from build123d import *

# Parameters (mm, degrees)
SKETCH1_R           = 2
BOSS_EXTRUDE1_DEPTH = 5
SKETCH2_R           = 4
CUT_EXTRUDE1_DEPTH  = 2
SKETCH3_R           = 11
SKETCH3_R_2         = 1.901621635
BOSS_EXTRUDE2_DEPTH = 12


with BuildPart() as part:
    # Sketch1 → Boss-Extrude1 (new body)
    with BuildSketch(Plane(origin=(0, 0, 0), x_dir=(1, 0, 0), z_dir=(0, 1, 0))):
        Polygon((0, 49), (0, 0), (49, 0), (49, 34), (34, 34), (34, 49), align=None)
        with Locations((15, 10.96347032)):
            Circle(SKETCH1_R, mode=Mode.SUBTRACT)
        with Locations((15, 25.96347032)):
            Circle(SKETCH1_R, mode=Mode.SUBTRACT)
        with Locations((15, 40.96347032)):
            Circle(SKETCH1_R, mode=Mode.SUBTRACT)
    extrude(amount=BOSS_EXTRUDE1_DEPTH)

    # Sketch2 → Cut-Extrude1 (cut)
    with BuildSketch(Plane(origin=(0, 5, 0), x_dir=(1, 0, 0), z_dir=(0, 1, 0))):
        with Locations((15, 40.96347032)):
            Circle(SKETCH2_R)
        with Locations((15, 10.96347032)):
            Circle(SKETCH2_R)
    extrude(amount=-CUT_EXTRUDE1_DEPTH, mode=Mode.SUBTRACT)

    # Sketch3 → Boss-Extrude2 (add)
    with BuildSketch(Plane(origin=(0, 5, 0), x_dir=(1, 0, 0), z_dir=(0, 1, 0))):
        with Locations((15, 25.96347032)):
            Circle(SKETCH3_R)
        with Locations((15, 25.96347032)):
            Circle(SKETCH3_R_2, mode=Mode.SUBTRACT)
    extrude(amount=BOSS_EXTRUDE2_DEPTH)


solid = part.part
The model under review builds one solid part; all positions refer to its coordinate system, in mm. A direction names the side the tool comes from. Round coordinates to 2 decimals unless told otherwise and drop trailing zeros. Order: outer loops, then holes, each group sorted by start corner. A loop starts at its lowest first (then second) coordinate and runs counter-clockwise, first axis right, second up. Notation, with made-up numbers: (-22.5, 78.5) -> (11.5, 78.5) arc R21 ccw to (11.5, 102.5) -> close; hole circle Ø11 at (62, -21.75). An arc over 180 degrees is marked (long way). Use CSV: the item, a comma, the result in double quotes. Start each with the question number.
(1) Wall thickness on probe 1 along Z at (x, y) = (15, 3.6); probe 2 along Z at (x, y) = (15, 1.2); probe 3 along Z at (x, y) = (15, 13): over which ranges is each line inside the solid? List them lowest first. Write a range as from..to.
(2) Consider section D-D on z = -36. Write out the cut boundary in (x, y), and give its area (3 significant figures).
(3) Consider section B-B on z = -14. Write out the cut boundary in (x, y).
(4) Mouldability with a two-part tool opening along Z and no side actions: class faces 5 (the face through (17.3, 17, -26.1)), 6 (the face through (24, 2, 0)), 7 (the face through (13, 3, -10)), 8 (the face through (14.74, 1.479, -42.946)) as pulls with the +Z half, pulls with the -Z half, needs draft (parallel to the pull), parting line crosses it, or undercut.
(5) Insertion check: pin 1 (1.5 mm diameter, centred on y = 2.5, z = -41.5, fed in from +X); pin 2 (9 mm diameter, centred on x = 14, z = -42.5, fed in from +Y); pin 3 (4 mm diameter, centred on x = 39.5, y = 2, fed in from -Z). Each pin has a flat end and moves straight along its axis. Give the tip position at first contact, or say it passes through.
(6) Consider section C-C on x = 40.5. Write out the cut boundary in (y, z), and give its area (3 significant figures).
(7) Consider section A-A on x = 14. State how many separate pieces and enclosed holes the cut face has, and give its area (3 significant figures).
(8) Tool access review of faces 1 (the face through (42, 2, -34)), 2 (the face through (14.74, 2.465, -27.946)), 3 (the face through (13.53, 1.48, -12.32)), 4 (the face through (14.48, 4.01, -44.93)): name each direction out of +Z, -Z, +X, -X, +Y, -Y from which nothing blocks a thin tool from reaching the whole face with its end or side.
Responses:
1,probe 1,"-49..-44.96, -36.96..-27.96, -23.96..-14.96, -6.96..0"
1,probe 2,"-49..-42.96, -38.96..-27.96, -23.96..-12.96, -8.96..0"
1,probe 3,"-36.96..-27.87, -24.06..-14.96"
2,outline,"(0, 0) -> (34, 0) -> (34, 5) -> (19.5, 5) -> (19.5, 17) -> (10.5, 17) -> (10.5, 5) -> (0, 5) -> close"
2,area,"278 mm²"
3,outline,"(0, 0) -> (49, 0) -> (49, 5) -> (17.6, 5) -> (17.6, 3) -> (12.4, 3) -> (12.4, 5) -> (0, 5) -> close"
4,face 5,"needs draft"
4,face 6,"pulls with the +Z half"
4,face 7,"undercut"
4,face 8,"undercut"
5,pin 1,"x = 34"
5,pin 2,"y = 5"
5,pin 3,"z = -34"
6,outline,"(0, -34) -> (5, -34) -> (5, 0) -> (0, 0) -> close"
6,area,"170 mm²"
7,separate pieces,"4"
7,enclosed holes,"0"
7,area,"400 mm²"
8,face 1,"-Z, +X, +Y, -Y"
8,face 2,"-Y"
8,face 3,"+Y, -Y"
8,face 4,"+Y"
